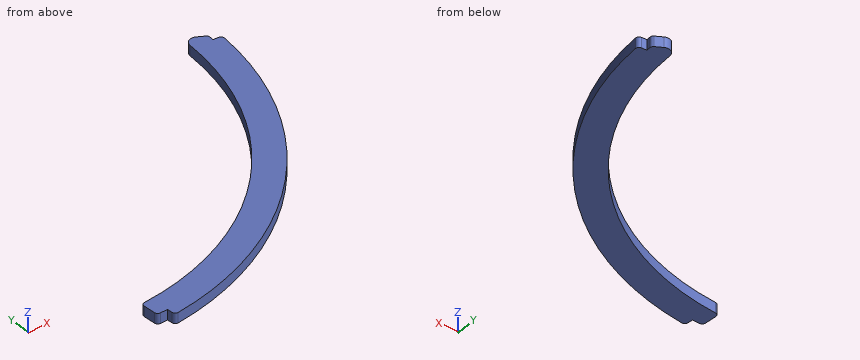
Autodesk Inventor part; units mm, degrees
ref_plane "YZ Plane" through (0, 0, 0) normal (1, 0, 0) x (0, 1, 0)
ref_plane "XZ Plane" through (0, 0, 0) normal (0, 1, 0) x (-1, 0, 0)
ref_plane "XY Plane" through (0, 0, 0) normal (0, 0, 1) x (1, 0, 0)
sketch "Sketch1" plane through (0, 0, 0) normal (0, 0, 1) x (1, 0, 0)
  arc A0 (5.6926, -80.7997) -> (80.8293, -5.2553) centre (0, 0) ccw
  arc A1 (2.1409, -72.9686) -> (72.998, -0.5377) centre (0, 0) ccw
  line L0 (72.998, -0.5377) -> (80.8095, -0.5953) construction
  line L1 (0, 0) -> (0, 0) construction
  line L2 (2.1409, -72.9686) -> (2.5169, -78.3059)
  line L3 (2.5169, -78.3059) -> (5.5169, -78.3059)
  line L4 (5.5169, -78.3059) -> (5.6926, -80.7997)
  line L5 (78.412, -3.7169) -> (72.998, -0.5377)
  line L6 (78.3059, -5.5169) -> (80.7997, -5.6926)
  arc A2 (78.3059, -5.5169) -> (78.412, -3.7169) centre (0, 0) ccw
  line L7 (0, 0) -> (0, -120.2528) construction
  line L8 (0, 0) -> (5.9355, -84.2471) construction
  line L9 (0, 0) -> (88.2589, 0) construction
  line L10 (0, 0) -> (93.5685, -6.5922) construction
  line L11 (72.998, -0.5377) -> (0, 0) construction
  dimension "d0" = 162
  dimension "d1" = 146
  dimension "d38" = 2.5
  dimension "d39" = 3
  dimension "d40" = 30
  dimension "d52" = 78.5
  dimension "d53" = 1.8
  dimension "d55" = 4.03
  dimension "d57" = 4.03
extrude "Extrusion1" add sketch "Sketch1" along normal blind 3
fillet "Fillet6" radius 2 1 edges at (72.998, -0.5377, 1.5)
sketch "Sketch5" plane through (0, 0, 3) normal (0, 0, 1) x (1, 0, 0)
  line L0 (10.4211, -74.15) -> (12.817, -75.9554)
  line L1 (12.817, -75.9554) -> (11.0116, -78.3513)
  line L2 (11.0116, -78.3513) -> (8.6157, -76.5459)
  line L3 (8.6157, -76.5459) -> (10.4211, -74.15)
  line L4 (0, 0) -> (11.0116, -78.3513) construction
  line L5 (12.817, -75.9554) -> (8.6157, -76.5459) construction
  line L6 (0, 0) -> (0, -125.3413) construction
  line L7 (15.0785, -75.539) -> (16.6742, -72.9985)
  line L8 (16.6742, -72.9985) -> (19.2146, -74.5942)
  line L9 (19.2146, -74.5942) -> (17.619, -77.1347)
  line L10 (17.619, -77.1347) -> (15.0785, -75.539)
  line L11 (21.4327, -73.9874) -> (22.8071, -71.3208)
  line L12 (22.8071, -71.3208) -> (25.4737, -72.6952)
  line L13 (25.4737, -72.6952) -> (24.0993, -75.3618)
  line L14 (24.0993, -75.3618) -> (21.4327, -73.9874)
  line L15 (27.6323, -71.9024) -> (28.7755, -69.1288)
  line L16 (28.7755, -69.1288) -> (31.5492, -70.272)
  line L17 (31.5492, -70.272) -> (30.406, -73.0456)
  line L18 (30.406, -73.0456) -> (27.6323, -71.9024)
  line L19 (33.6327, -69.2989) -> (34.5365, -66.4383)
  line L20 (34.5365, -66.4383) -> (37.3971, -67.3421)
  line L21 (37.3971, -67.3421) -> (36.4933, -70.2027)
  line L22 (36.4933, -70.2027) -> (33.6327, -69.2989)
  line L23 (39.3906, -66.1958) -> (40.0484, -63.2688)
  line L24 (40.0484, -63.2688) -> (42.9754, -63.9266)
  line L25 (42.9754, -63.9266) -> (42.3176, -66.8536)
  line L26 (42.3176, -66.8536) -> (39.3906, -66.1958)
  line L27 (44.8644, -62.6154) -> (45.2716, -59.6431)
  line L28 (45.2716, -59.6431) -> (48.2438, -60.0503)
  line L29 (48.2438, -60.0503) -> (47.8367, -63.0225)
  line L30 (47.8367, -63.0225) -> (44.8644, -62.6154)
  line L31 (50.0148, -58.5834) -> (50.1683, -55.5874)
  line L32 (50.1683, -55.5874) -> (53.1644, -55.7409)
  line L33 (53.1644, -55.7409) -> (53.0109, -58.737)
  line L34 (53.0109, -58.737) -> (50.0148, -58.5834)
  line L35 (54.8046, -54.1291) -> (54.7033, -51.1308)
  line L36 (54.7033, -51.1308) -> (57.7016, -51.0296)
  line L37 (57.7016, -51.0296) -> (57.8028, -54.0279)
  line L38 (57.8028, -54.0279) -> (54.8046, -54.1291)
  line L39 (59.1991, -49.2845) -> (58.8439, -46.3056)
  line L40 (58.8439, -46.3056) -> (61.8228, -45.9504)
  line L41 (61.8228, -45.9504) -> (62.178, -48.9293)
  line L42 (62.178, -48.9293) -> (59.1991, -49.2845)
  line L43 (63.1669, -44.0845) -> (62.5602, -41.1465)
  line L44 (62.5602, -41.1465) -> (65.4982, -40.5399)
  line L45 (65.4982, -40.5399) -> (66.1049, -43.4779)
  line L46 (66.1049, -43.4779) -> (63.1669, -44.0845)
  line L47 (66.6792, -38.5667) -> (65.8254, -35.6907)
  line L48 (65.8254, -35.6907) -> (68.7014, -34.837)
  line L49 (68.7014, -34.837) -> (69.5551, -37.713)
  line L50 (69.5551, -37.713) -> (66.6792, -38.5667)
  line L51 (69.7107, -32.7708) -> (68.616, -29.9776)
  line L52 (68.616, -29.9776) -> (71.4092, -28.883)
  line L53 (71.4092, -28.883) -> (72.5038, -31.6761)
  line L54 (72.5038, -31.6761) -> (69.7107, -32.7708)
  line L55 (72.2395, -26.7386) -> (70.9119, -24.0483)
  line L56 (70.9119, -24.0483) -> (73.6021, -22.7207)
  line L57 (73.6021, -22.7207) -> (74.9298, -25.4109)
  line L58 (74.9298, -25.4109) -> (72.2395, -26.7386)
  line L59 (74.2475, -20.5136) -> (72.6964, -17.9457)
  line L60 (72.6964, -17.9457) -> (75.2643, -16.3946)
  line L61 (75.2643, -16.3946) -> (76.8154, -18.9625)
  line L62 (76.8154, -18.9625) -> (74.2475, -20.5136)
  line L63 (75.7202, -14.1407) -> (73.9568, -11.7136)
  line L64 (73.9568, -11.7136) -> (76.3838, -9.9503)
  line L65 (76.3838, -9.9503) -> (78.1472, -12.3773)
  line L66 (78.1472, -12.3773) -> (75.7202, -14.1407)
  line L67 (73.9568, -11.7136) -> (78.1472, -12.3773) construction
  point P0 (10.7163, -76.2506)
  dimension "d43" = 3
  dimension "d44" = 77
  dimension "d45" = 8
  dimension "d48" = 73
  dimension "d58" = 73
extrude "Extrusion5" [suppressed]
fillet "Fillet7" radius 1 5 edges at (78.412, -3.7169, 1.5) (80.7997, -5.6926, 1.5) (5.6926, -80.7997, 1.5) (2.1409, -72.9686, 1.5) (2.5169, -78.3059, 1.5)
sketch "Sketch3" plane through (0, 0, 3) normal (0, 0, 1) x (1, 0, 0)
  line L0 (10, -73.0753) -> (2.1409, -73.0753)
  circle A0 centre (3.5, -73.0753) radius 1.5
  line L1 (2.1409, -72.9686) -> (2.7074, -81.01) construction
  line L2 (2, -77.0253) -> (11.8753, -77.0253) construction
  ellipse E0 centre (3.5, -81.0253) end of major axis (5, -81.0253) minor radius 0.75
  point P0 (0, 0)
  point P1 (5.6926, -80.7997)
  point P2 (2, -73.0753)
  point P3 (5, -73.0753)
  dimension "d15" = 3
  dimension "d16" = 1.5
  dimension "d20" = 0.75
  dimension "d21" = 1.5
  dimension "d22" = 4
sketch "Sketch4" plane through (0, 0, 3) normal (0, 0, 1) x (1, 0, 0)
  line L0 (80.9861, -1.5) -> (70.9842, -1.5)
  line L1 (80.9861, -1.5) -> (78.9861, -1.5)
  line L2 (78.9861, -4) -> (80.9012, -4)
  arc A0 (4.9576, -80.8481) -> (80.9861, -1.5) centre (0, 0) ccw
  arc A1 (80.9012, -4) -> (80.9861, -1.5) centre (0, 0) ccw
  line L3 (78.9861, -1.5) -> (78.9861, -4)
  line L4 (74.2542, -1.5) -> (70.9842, -1.5)
  arc A2 (10.8472, -70.1665) -> (70.9842, -1.5) centre (0, 0) ccw
  arc A3 (70.8727, -4.25) -> (70.9842, -1.5) centre (0, 0) ccw
  line L5 (70.8727, -4.25) -> (74.2542, -4.25)
  line L6 (74.2542, -4.25) -> (74.2542, -1.5)
  point P0 (10, -70.2922)
  dimension "d25" = 2.5
  dimension "d30" = 2
  dimension "d31" = 2.75
  dimension "d32" = 3.27
properties part number "shim_cartridge_V4"
Verification items for the finished model (mm, model axes). Coordinates: 2 decimals unless noted, no trailing zeros. Order: outer loops, then holes, each group sorted by start corner. A loop starts at its lowest first (then second) coordinate and runs counter-clockwise, first axis right, second up. Notation, with made-up numbers: M 29.25,-9 L 55.25,-9 A27 cw 55.25,27 Z; hole C 54,58 d11. An arc over 180 degrees is marked long. One line per item, written item: value. Start each with the question number.
Item 1: Scan lines: probe 1 along X at (y, z) = (-10, 1.2); probe 2 along X at (y, z) = (-47, 0.3); probe 3 along Y at (x, z) = (12, 0.6). Record each from-to range of solid material in increasing order.
Item 2: Sectioned sample at B-B (x = 65). Enter the section's corners in (y, z).
Item 3: Sectioned sample at C-C (y = -13). Enter the section's corners in (x, z).
Item 4: Sectioned sample at A-A (z = 2.4). Enter the section's corners in (x, y).
Item 5: Gauge pin test, flat end, axial feed: pin 1 (6 mm diameter, centred on x = 38.5, y = -59, fed in from +Z). Record the tip position at first contact, or that the pin passes through.
Conclusion:
1. probe 1: x = 72.31 to 80.38
1. probe 2: x = 55.86 to 65.97
1. probe 3: y = -80.11 to -72.01
2. outline: M -48.33,0 L -33.23,0 L -33.23,3 L -48.33,3 Z
3. outline: M 71.83,0 L 79.95,0 L 79.95,3 L 71.83,3 Z
4. outline: M 2.21,-74 L 2.45,-77.38 A1 ccw 3.45,-78.31 L 5.52,-78.31 L 5.62,-79.8 A1 ccw 6.7,-80.72 A81 ccw 80.72,-6.7 A1 ccw 79.8,-5.62 L 78.31,-5.52 A78.84 ccw 78.38,-4.33 A1 ccw 77.89,-3.41 L 75.91,-2.25 A2 ccw 72.9,-3.86 A73 cw 3.17,-72.93 A1 ccw Z
5. pin 1: stops at z = 3
